CAD build for the part. Positions are in the model's coordinates, mm. A direction names the side the tool comes from. Coordinates: 2 decimals unless noted, no trailing zeros. Loops run counter-clockwise (first coordinate to the right, second up) from the corner with the lowest first, then second, coordinate; pieces in that order, holes last. Notation, with made-up numbers: (-2.75, 56.5) -> (18.25, 56.5) arc R13 cw to (18.25, 60.5) -> close; hole circle Ø2 at (79, -25). An arc over 180 degrees is marked (long way). Return JSON: item names as keys, results as strings. Group by question number.
(1) Probe L1, parallel to X at y = -2.25, z = 0; L2, parallel to Y at x = 7.5, z = -14.5; L3, parallel to Z at x = -8, y = -1.5. List the from-to ranges inside material, lowest first.
(2) Mould opens along Z. For faces 5 (the face through (26.92, 0.76, -26.82)), 6 (the face through (0, 1, 28)), 7 (the face through (24.37, 0.74, -20.13)), 8 (the face through (0, 1.5, 0)) say: pulls with the +Z half, pulls with the -Z half, needs draft (parallel to the pull), parting line crosses it, or undercut.
(3) Tool access for faces 1 (the face through (23.479, 0.76, 25.722)), 2 (the face through (-20.06, 0.76, -24.3)), 3 (the face through (2.17, -4.44, 9.76)), 4 (the face through (20.13, 0.74, 24.37)): list every direction of +Z, -Z, +X, -X, +Y, -Y with a clear straight run to the whole face (end or side of a thin tool).
(4) Saw through at D-D on x = -11.5. Write the cut outline in (y, z), then the cut area to 3 significant figures.
(5) Saw through at C-C on y = -1. Write the cut outline in (x, z).
(6) Saw through at A-A on x = 0. Write the cut outline in (y, z), then the cut area to 3 significant figures.
(7) Flat gauge pins, fed straight in: pin 1 Ø1 at (y, z) = (-7.5, 2.5) entering from -X; pin 2 Ø3 at (y, z) = (0, -10) entering from +X; pin 3 Ø6 at (x, z) = (3.5, -2) entering from -Y; pin 4 Ø3.5 at (x, z) = (-24.75, 24.75) entering from +Y. Where does each tip first touch, or does it go through?
(8) Saw through at B-B on z = 0. Write the cut outline in (x, y).
```python
from build123d import *

# Parameters (mm, degrees)
SKETCH1_R                = 1.6
BOSS_EXTRUDE1_DEPTH      = 1.5
FILLET1_R                = 2
SKETCH2_R                = 4
BOSS_EXTRUDE2_DEPTH      = 5
SKETCH5_R                = 13.8
BOSS_EXTRUDE4_DEPTH      = 3
BOSS_EXTRUDE4_DEPTH_BACK = 5
SKETCH6_R                = 10
CUT_EXTRUDE2_DEPTH       = 8
SKETCH3_R                = 1.6
BOSS_EXTRUDE5_DEPTH      = 1.5
SKETCH7_R                = 13.8
SKETCH7_R_2              = 10
BOSS_EXTRUDE6_DEPTH      = 5
SKETCH8_R                = 13.8
CUT_EXTRUDE3_DEPTH       = 3
SKETCH9_R                = 13.8
CUT_EXTRUDE4_DEPTH       = 1
SKETCH10_R               = 28
BOSS_EXTRUDE7_DEPTH      = 1.5


with BuildPart() as part:
    # Sketch1 → Boss-Extrude1 (new body)
    with BuildSketch(Plane(origin=(0, 0, 0), x_dir=(1, 0, 0), z_dir=(0, 1, 0))):
        with BuildLine():
            Line((-23.334523779, -19.091883092), (-20.383302711, -16.140662024))
            ThreePointArc((-20.383302711, -16.140662024), (-26, 0), (-20.383302711, 16.140662024))
            Line((-20.383302711, 16.140662024), (-23.334523779, 19.091883092))
            ThreePointArc((-23.334523779, 19.091883092), (-23.334523779, 23.334523779), (-19.091883092, 23.334523779))
            Line((-19.091883092, 23.334523779), (-16.140662024, 20.383302711))
            ThreePointArc((-16.140662024, 20.383302711), (0, 26), (16.140662024, 20.383302711))
            Line((16.140662024, 20.383302711), (19.091883092, 23.334523779))
            ThreePointArc((19.091883092, 23.334523779), (23.334523779, 23.334523779), (23.334523779, 19.091883092))
            Line((23.334523779, 19.091883092), (20.383302711, 16.140662024))
            ThreePointArc((20.383302711, 16.140662024), (26, 0), (20.383302711, -16.140662024))
            Line((20.383302711, -16.140662024), (23.334523779, -19.091883092))
            ThreePointArc((23.334523779, -19.091883092), (23.334523779, -23.334523779), (19.091883092, -23.334523779))
            Line((19.091883092, -23.334523779), (16.140662024, -20.383302711))
            ThreePointArc((16.140662024, -20.383302711), (0, -26), (-16.140662024, -20.383302711))
            Line((-16.140662024, -20.383302711), (-19.091883092, -23.334523779))
            ThreePointArc((-19.091883092, -23.334523779), (-23.334523779, -23.334523779), (-23.334523779, -19.091883092))
        make_face()
        with Locations((-21.213203436, 21.213203436)):
            Circle(SKETCH1_R, mode=Mode.SUBTRACT)
        with Locations((21.213203436, 21.213203436)):
            Circle(SKETCH1_R, mode=Mode.SUBTRACT)
        with Locations((-21.213203436, -21.213203436)):
            Circle(SKETCH1_R, mode=Mode.SUBTRACT)
        with Locations((21.213203436, -21.213203436)):
            Circle(SKETCH1_R, mode=Mode.SUBTRACT)
    extrude(amount=BOSS_EXTRUDE1_DEPTH)

    # Fillet1
    fillet1_edges = [part.edges().sort_by_distance(p)[0] for p in [
        (-20.383302711, 0.75, -16.140662024),
        (-16.140662024, 0.75, -20.383302711),
        (16.140662024, 0.75, -20.383302711),
        (20.383302711, 0.75, -16.140662024),
        (20.383302711, 0.75, 16.140662024),
        (16.140662024, 0.75, 20.383302711),
        (-16.140662024, 0.75, 20.383302711),
    ]]
    fillet(fillet1_edges, radius=FILLET1_R)

    # Sketch2 → Boss-Extrude2 (add)
    with BuildSketch(Plane(origin=(0, 0, 0), x_dir=(-1, 0, 0), z_dir=(0, -1, 0))):
        Circle(SKETCH2_R)
    extrude(amount=BOSS_EXTRUDE2_DEPTH)

    # Sketch5 → Boss-Extrude4 (add, two sides)
    with BuildSketch(Plane(origin=(0, -5, 0), x_dir=(-1, 0, 0), z_dir=(0, -1, 0))) as boss_extrude4_sk:
        Circle(SKETCH5_R)
    extrude(amount=BOSS_EXTRUDE4_DEPTH)
    extrude(boss_extrude4_sk.sketch, amount=-BOSS_EXTRUDE4_DEPTH_BACK)

    # Sketch6 → Cut-Extrude2 (cut)
    with BuildSketch(Plane(origin=(0, -8, 0), x_dir=(-1, 0, 0), z_dir=(0, -1, 0))):
        Circle(SKETCH6_R)
    extrude(amount=-CUT_EXTRUDE2_DEPTH, mode=Mode.SUBTRACT)

    # Sketch3 → Boss-Extrude5 (add)
    with BuildSketch(Plane(origin=(0, 1.5, 0), x_dir=(1, 0, 0), z_dir=(0, 1, 0))):
        with BuildLine():
            Line((-26.870057685, 22.627416998), (-19.914697313, 15.672056626))
            Line((-19.914697313, 15.672056626), (-15.672056626, 19.914697313))
            Line((-15.672056626, 19.914697313), (-22.627416998, 26.870057685))
            ThreePointArc((-22.627416998, 26.870057685), (-26.870057685, 26.870057685), (-26.870057685, 22.627416998))
        make_face()
        with Locations((-24.748737342, 24.748737342)):
            Circle(SKETCH3_R, mode=Mode.SUBTRACT)
        with BuildLine():
            Line((15.672056626, 19.914697313), (19.914697313, 15.672056626))
            Line((19.914697313, 15.672056626), (26.870057685, 22.627416998))
            ThreePointArc((26.870057685, 22.627416998), (26.870057685, 26.870057685), (22.627416998, 26.870057685))
            Line((22.627416998, 26.870057685), (15.672056626, 19.914697313))
        make_face()
        with Locations((24.748737342, 24.748737342)):
            Circle(SKETCH3_R, mode=Mode.SUBTRACT)
        with BuildLine():
            Line((26.870057685, -22.627416998), (19.914697313, -15.672056626))
            Line((19.914697313, -15.672056626), (15.672056626, -19.914697313))
            Line((15.672056626, -19.914697313), (22.627416998, -26.870057685))
            ThreePointArc((22.627416998, -26.870057685), (26.870057685, -26.870057685), (26.870057685, -22.627416998))
        make_face()
        with Locations((24.748737342, -24.748737342)):
            Circle(SKETCH3_R, mode=Mode.SUBTRACT)
        with BuildLine():
            Line((-15.672056626, -19.914697313), (-19.914697313, -15.672056626))
            Line((-19.914697313, -15.672056626), (-26.870057685, -22.627416998))
            ThreePointArc((-26.870057685, -22.627416998), (-26.870057685, -26.870057685), (-22.627416998, -26.870057685))
            Line((-22.627416998, -26.870057685), (-15.672056626, -19.914697313))
        make_face()
        with Locations((-24.748737342, -24.748737342)):
            Circle(SKETCH3_R, mode=Mode.SUBTRACT)
    extrude(amount=-BOSS_EXTRUDE5_DEPTH)

    # Sketch7 → Boss-Extrude6 (add)
    with BuildSketch(Plane(origin=(0, -8, 0), x_dir=(-1, 0, 0), z_dir=(0, -1, 0))):
        Circle(SKETCH7_R)
        Circle(SKETCH7_R_2, mode=Mode.SUBTRACT)
    extrude(amount=BOSS_EXTRUDE6_DEPTH)

    # Sketch8 → Cut-Extrude3 (cut)
    with BuildSketch(Plane(origin=(0, -13, 0), x_dir=(-1, 0, 0), z_dir=(0, -1, 0))):
        Circle(SKETCH8_R)
    extrude(amount=-CUT_EXTRUDE3_DEPTH, mode=Mode.SUBTRACT)

    # Sketch9 → Cut-Extrude4 (cut)
    with BuildSketch(Plane(origin=(0, -10, 0), x_dir=(-1, 0, 0), z_dir=(0, -1, 0))):
        Circle(SKETCH9_R)
    extrude(amount=-CUT_EXTRUDE4_DEPTH, mode=Mode.SUBTRACT)

    # Sketch10 → Boss-Extrude7 (add)
    with BuildSketch(Plane(origin=(0, 1.5, 0), x_dir=(1, 0, 0), z_dir=(0, 1, 0))):
        Circle(SKETCH10_R)
    extrude(amount=-BOSS_EXTRUDE7_DEPTH)


solid = part.part
```
Geometry results:
{
 "1": {"L1": "-13.8 to -10, 10 to 13.8", "L2": "0 to 1.5", "L3": "-11.24 to -6, 6 to 11.24"},
 "2": {"face 5": "undercut", "face 6": "pulls with the +Z half", "face 7": "undercut", "face 8": "needs draft"},
 "3": {"face 1": "+Y, -Y", "face 2": "-Z, +Y, -Y", "face 3": "-Y", "face 4": "+Z, +Y, -Y"},
 "4": {"outline": "(-9, -7.63) -> (0, -7.63) -> (0, -25.53) -> (1.5, -25.53) -> (1.5, 25.53) -> (0, 25.53) -> (0, 7.63) -> (-9, 7.63) -> close", "area": "214 mm²"},
 "5": {"outline": "circle Ø27.6 at (0, 0); hole circle Ø20 at (0, 0)"},
 "6": {"outline": "(-9, -13.8) -> (0, -13.8) -> (0, -28) -> (1.5, -28) -> (1.5, 28) -> (0, 28) -> (0, 13.8) -> (-9, 13.8) -> (-9, 10) -> (0, 10) -> (0, -10) -> (-9, -10) -> close", "area": "152 mm²"},
 "7": {"pin 1": "x = -13.65", "pin 2": "x = 26.68", "pin 3": "y = 0", "pin 4": "y = 1.5"},
 "8": {"outline": "(-28, 0) -> (-13.8, 0) -> (-13.8, -9) -> (-10, -9) -> (-10, 0) -> (10, 0) -> (10, -9) -> (13.8, -9) -> (13.8, 0) -> (28, 0) -> (28, 1.5) -> (-28, 1.5) -> close"}
}
